Autodesk Inventor part; units mm, degrees
ref_plane "YZ Plane" through (0, 0, 0) normal (1, 0, 0) x (0, 1, 0)
ref_plane "XZ Plane" through (0, 0, 0) normal (0, 1, 0) x (-1, 0, 0)
ref_plane "XY Plane" through (0, 0, 0) normal (0, 0, 1) x (1, 0, 0)
sketch "Boceto1" plane through (0, 0, 0) normal (0, 1, 0) x (-1, 0, 0)
  line L0 (-20, 15) -> (20, 15)
  line L1 (25, 10) -> (25, -10)
  line L2 (20, -15) -> (-20, -15)
  line L3 (-25, -10) -> (-25, 10)
  line L4 (-25, 15) -> (25, -15) construction
  line L5 (25, 15) -> (-25, -15) construction
  line L6 (21, -11) -> (21, 11)
  line L7 (21, 11) -> (-19, 11)
  line L8 (-21, 9) -> (-21, -9)
  line L9 (-19, -11) -> (21, -11)
  arc A0 (25, 10) -> (20, 15) centre (20, 10) ccw
  arc A1 (20, -15) -> (25, -10) centre (20, -10) ccw
  arc A2 (-25, -10) -> (-20, -15) centre (-20, -10) ccw
  arc A3 (-20, 15) -> (-25, 10) centre (-20, 10) ccw
  arc A4 (-19, 11) -> (-21, 9) centre (-19, 9) ccw
  arc A5 (-21, -9) -> (-19, -11) centre (-19, -9) ccw
  point P0 (0, 0)
  dimension "d0" = 50
  dimension "d1" = 30
  dimension "d2" = 4
  dimension "d3" = 5
  dimension "d4" = 2
extrude "Extrusión1" add sketch "Boceto1" along normal blind 2 contours L0 A0 L1 A1 L2 A2 L3 A3 | L9 A5 L8 A4 L7 L6
extrude "Extrusión2" add sketch "Boceto1" against normal blind 5
sketch "Boceto3" plane through (20, 2, -15) normal (0, 0, -1) x (-1, 0, 0)
  line L0 (1, -2) -> (41, -2)
  line L1 (1, -2) -> (1, -7)
  line L2 (41, -7) -> (1, -7)
  line L3 (41, -2) -> (41, -7)
  line L4 (41, -4.5) -> (38, -4.5)
  circle A0 centre (38, -4.5) radius 2.5
  circle A1 centre (38, -4.5) radius 1.25
  point P0 (20, -2)
  dimension "d9" = 3
  dimension "d10" = 2.5
extrude "Extrusión3" cut sketch "Boceto3" against normal through all contours A1
fillet "Empalme1" radius 2 8 edges at (-23.5355, -5, -13.5355) (0, -5, -15) (23.5355, -5, -13.5355) (25, -5, 0) (23.5355, -5, 13.5355) (0, -5, 15) (-23.5355, -5, 13.5355) (-25, -5, 0)
fillet "Empalme2" radius 0.5 6 edges at (20.4142, 0, 10.4142) (21, 0, 0) (20.4142, 0, -10.4142) (-1, 0, -11) (-1, 0, 11) (-21, 0, 0)
properties part number "Base2"
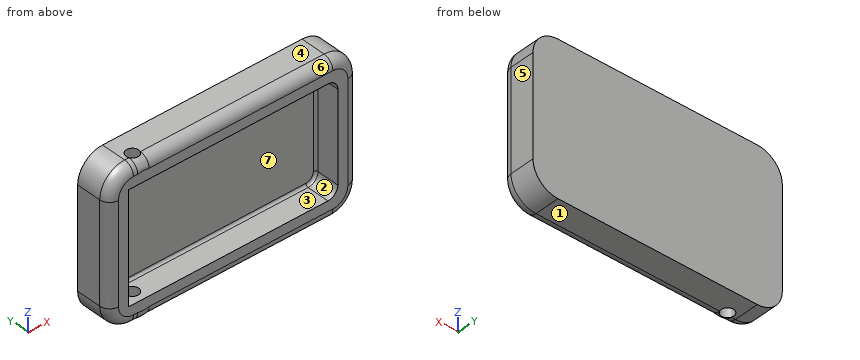
Could you check a few things on this model? Use its own coordinates, in mm. Face numbers are marked on the shaded views. A direction names the side the tool comes from. Give positions to 0.01 mm unless a question says otherwise; leave off trailing zeros. Loops run counter-clockwise (first coordinate to the right, second up) from the corner with the lowest first, then second, coordinate; pieces in that order, holes last. Notation, with made-up numbers: (72.25, -21) - (92.25, -21) arc R18 cw to (92.25, -5) - close; hole circle Ø11 at (20.5, 31). An arc over 180 degrees is marked (long way). Use one line per item in the form item = value.
1. I want a section at A-A (y = -2.5). Please give me the cut outline in (x, z), and give its area (3 significant figures).
Response values:
outline = (-25, -10) arc R5 ccw to (-20, -15) - (-19.25, -15) - (-19.25, -11) - (-21, -11) - (-21, 11) - (-19.25, 11) - (-19.25, 15) - (-20, 15) arc R5 ccw to (-25, 10) - close; (-16.75, -15) - (20, -15) arc R5 ccw to (25, -10) - (25, 10) arc R5 ccw to (20, 15) - (-16.75, 15) - (-16.75, 11) - (19, 11) arc R2 cw to (21, 9) - (21, -9) arc R2 cw to (19, -11) - (-16.75, -11) - close
area = 536 mm²
2. I'm going to push flat-ended pins straight in: pin 1 Ø2 at (x, y) = (-18, -2.5) entering from -Z (3 decimals); pin 2 Ø4 at (x, z) = (-1.5, 3.5) entering from -Y. Where does each tip first touch, or does it pass through?
Response values:
pin_1 = through
pin_2 = 0
3. Thinking about a two-plate mould opening in Z: for the marked faces 1, 2, 3 and 4, which applies, released by +Z, released by -Z, zero draft, split by the parting line, or undercut?
Response values:
face_1 = released by -Z
face_2 = undercut
face_3 = undercut
face_4 = released by +Z
4. I want a section at C-C (x = -14.5). Please give me the cut outline in (y, z).
Response values:
outline = (-5, -13) arc R2 ccw to (-3, -15) - (2, -15) - (2, 15) - (-3, 15) arc R2 ccw to (-5, 13) - (-5, 11) - (-0.5, 11) arc R0.5 cw to (0, 10.5) - (0, -10.5) arc R0.5 cw to (-0.5, -11) - (-5, -11) - close
5. I need wall thicknesses on probe 1 along X at (y, z) = (-3, -2); probe 2 along Z at (x, y) = (-11, -3); probe 3 along Y at (x, z) = (-18, -13.2). Which ranges of each line are inside material? Lowest first, please.
Response values:
probe_1 = -25 to -21, 21 to 25
probe_2 = -15 to -11, 11 to 15
probe_3 = -5 to -3.75, -1.25 to 2
6. I want a section at B-B (z = 7). Please give me the cut outline in (x, y), and give its area (3 significant figures).
Response values:
outline = (-25, -3) arc R2 ccw to (-23, -5) - (-21, -5) - (-21, -0.5) arc R0.5 cw to (-20.5, 0) - (20.5, 0) arc R0.5 cw to (21, -0.5) - (21, -5) - (23, -5) arc R2 ccw to (25, -3) - (25, 2) - (-25, 2) - close
area = 138 mm²
7. On a 3-axis mill with a long thin cutter (end or side, diameter ignored), from which of +Z, -Z, +X, -X, +Y, -Y can I reach the whole of each face in a straight line? I mean the marked faces 5, 6 and 7. Say none if no direction works.
Response values:
face_5 = +Z, -Z, +X, +Y, -Y
face_6 = +Z, +X, -Y
face_7 = -Y
